Autodesk Fusion 360 part; units mm, degrees
sketch "Sketch1" plane through (0, 0, 0) normal (0, 1, 0) x (1, 0, 0)
  line L0 (-5, -120) -> (5, -120)
  line L1 (5, -120) -> (5, 120)
  line L2 (5, 120) -> (-5, 120)
  line L3 (-5, 120) -> (-5, -120)
  circle A0 centre (0, -70) radius 3.5
  circle A1 centre (0, 50) radius 3.5
  dimension "d1" = 240
  dimension "d3" = 7
  dimension "d4" = 7
  dimension "d5" = 120
  dimension "d6" = 120
  dimension "d7" = 50
extrude "Extrude1" add sketch "Sketch1" along normal blind 2
Source: CAD feature listing. Evaluate the final solid. Frame: model axes, mm. Round coordinates to 2 decimals unless told otherwise and drop trailing zeros. Loops run counter-clockwise (first coordinate to the right, second up) from the corner with the lowest first, then second, coordinate; pieces in that order, holes last. Notation, with made-up numbers: (41.5, 18) - (85.5, 18) arc R20 cw to (85.5, 47) - close; hole circle Ø8 at (66.5, -37.75). An arc over 180 degrees is marked (long way). Write item = value, one per line. Start each with the question number.
(1) Section query B-B, the plane z = -50. Output: boundary loops of the cut face in (x, y).
(2) Section query C-C, the plane y = 1.1. Output: boundary loops of the cut face in (x, z), plus the area to 3 significant figures.
(3) Ray query, line 1 along Z through (x, y) = (0, 0.55); line 2 along X through (y, z) = (1.35, -50); line 3 along Z through (x, y) = (1.5, 1.1). Return the intervals inside material, ascending. Write a range as from..to.
(4) Section query A-A, the plane x = 0. Output: boundary loops of the cut face in (y, z), plus the area to 3 significant figures.
(5) Pull-direction query (Z, two-part tool) for faces 1 (the face through (-0.759, 0.986, 66.583)), 2 (the face through (0, 2, -2)); classes: +Z half, -Z half, draft (parallel to the pull), parting line (faces both ways), or undercut.
Conclusion:
q1.outline = (-5, 0) - (-3.5, 0) - (-3.5, 2) - (-5, 2) - close; (3.5, 0) - (5, 0) - (5, 2) - (3.5, 2) - close
q2.outline = (-5, -120) - (5, -120) - (5, 120) - (-5, 120) - close; hole circle Ø7 at (0, -50); hole circle Ø7 at (0, 70)
q2.area = 2,320 mm2
q3.line_1 = -120..-53.5, -46.5..66.5, 73.5..120
q3.line_2 = -5..-3.5, 3.5..5
q3.line_3 = -120..-53.16, -46.84..66.84, 73.16..120
q4.outline = (0, -120) - (2, -120) - (2, -53.5) - (0, -53.5) - close; (0, -46.5) - (2, -46.5) - (2, 66.5) - (0, 66.5) - close; (0, 73.5) - (2, 73.5) - (2, 120) - (0, 120) - close
q4.area = 452 mm2
q5.face_1 = undercut
q5.face_2 = draft
